Autodesk Inventor part; units mm, degrees
ref_plane "Plano de trabajo1" through (0, 0, 17.5) normal (0, 0, 1) x (1, 0, 0)
ref_plane "YZ Plane" through (0, 0, 0) normal (1, 0, 0) x (0, 1, 0)
ref_plane "XZ Plane" through (0, 0, 0) normal (0, 1, 0) x (-1, 0, 0)
sketch "Boceto1" plane through (0, 0, 0) normal (0, 1, 0) x (-1, 0, 0)
  circle A0 centre (0, 0) radius 17.5
  dimension "d0" = 35
extrude "Extrusión1" add sketch "Boceto1" along normal blind 805
shell "Vaciado1" thickness 2 removed faces 2 at (-4.3663, 0, -1.0762) at (-4.3663, 805, -1.0762)
ref_plane "Plano de trabajo1" through (0, 0, 17.5) normal (0, 0, 1) x (1, 0, 0)
sketch "Boceto2" plane through (0, 0, 17.5) normal (0, 0, 1) x (1, 0, 0)
  line L0 (0, 81.1949) -> (0, -92.1127) construction
  line L1 (-146.6766, 0) -> (158.2781, 0) construction
  circle A0 centre (0, 10) radius 4
  point P0 (0, 0)
  dimension "d5" = 8
  dimension "d6" = 10
extrude "Extrusión2" cut sketch "Boceto2" against normal blind 50
Build history of the part. All positions in model axes, mm. Round coordinates to 2 decimals unless told otherwise and drop trailing zeros. Write each loop counter-clockwise with the first axis right and the second up, starting at its lowest first coordinate (ties: lowest second). Pieces come first, ordered by that corner, then holes. Notation, with made-up numbers: M 10.25,-2 L 57.25,-2 A27 ccw 57.25,36 Z; hole C -28,27 d4. An arc over 180 degrees is marked long. Answer as a JSON object with one key per item and string values. Group by question number.
(1) Cut at A-A (z = 0). Give the cut face in (x, y), and give its area (3 significant figures).
(2) Flat gauge pins, fed straight in: pin 1 (18.5 mm diameter, centred on x = 0, z = 0, fed in from +Y); pin 2 (6 mm diameter, centred on y = 159.5, z = 11, fed in from -X); pin 3 (4 mm diameter, centred on x = -6.5, y = 191.5, fed in from -Z). Where does each tip first touch, or does it go through?
(3) Cut at C-C (y = 159.5). Give the cut face in (x, z), and give its area (3 significant figures).
(4) Cut at B-B (x = 10). Give the cut face in (y, z).
(5) Drill centre lines: L1, parallel to Y at x = 0, z = -16.1; L2, parallel to X at y = 440, z = 2; L3, parallel to Z at x = 0, y = 300. Where is each one in solid material? Low to high.
(6) Mould opens along X. For faces 1 (the cylindrical face through (13.887, 396.865, 10.648)), 2 (the cylindrical face through (2.018, 396.865, -15.368)), 3 (the flat face through (7, 805, -14)) say: pulls with the +X half, pulls with the -X half, needs draft (parallel to the pull), parting line crosses it, or undercut.
Responses:
{
 "1": {"outline": "M -17.5,0 L -15.5,0 L -15.5,805 L -17.5,805 Z; M 15.5,0 L 17.5,0 L 17.5,805 L 15.5,805 Z", "area": "3,220 mm2"},
 "2": {"pin 1": "passes through", "pin 2": "stops at x = -15.56", "pin 3": "stops at z = -16.91"},
 "3": {"outline": "C 0,0 d35; hole C 0,0 d31", "area": "207 mm2"},
 "4": {"outline": "M 0,-14.36 L 805,-14.36 L 805,-11.84 L 0,-11.84 Z; M 0,11.84 L 805,11.84 L 805,14.36 L 0,14.36 Z"},
 "5": {"L1": "y = 0 to 6, 14 to 805", "L2": "x = -17.39 to -15.37, 15.37 to 17.39", "L3": "z = -17.5 to -15.5, 15.5 to 17.5"},
 "6": {"face 1": "parting line crosses it", "face 2": "undercut", "face 3": "needs draft"}
}
